Here's how the part is built. I have some questions about the finished solid (model axes, mm). A direction names the side the tool comes from. Round coordinates to 2 decimals unless told otherwise and drop trailing zeros. Order: outer loops, then holes, each group sorted by start corner. A loop starts at its lowest first (then second) coordinate and runs counter-clockwise, first axis right, second up. Notation, with made-up numbers: M -27.5,-31.5 L 25.5,-31.5 A22 cw 25.5,-1.5 Z; hole C 1.25,13 d11. An arc over 180 degrees is marked long. Write item = value, one per line. Start each with the question number.
Item 1: We'd pull the mould along Y, two halves only. Please class faces 1 (the face through (20.95, 4.035, 18.483)), 2 (the face through (-16, -3.204, 11)), 3 (the face through (-28, -1, 23)): pulls with the +Y half, pulls with the -Y half, needs draft (parallel to the pull), parting line crosses it, or undercut.
Item 2: I'm going to push flat-ended pins straight in: P1, Ø2, axis at x = -27, z = 12.5, coming from the +Y side; P2, Ø2, axis at x = -16, y = -0.5, coming from the +Z side; P3, Ø1.5, axis at x = -19.5, z = 3.5, coming from the -Y side; P4, Ø1.5, axis at x = 14.5, z = 8.5, coming from the -Y side. Where does each tip first touch, or does it pass through?
Item 3: I want a section at C-C, the plane x = -19.5. List the corners of the cut face in (y, z) for me, plus the area to 3 significant figures.
Item 4: I want a section at A-A, the plane z = 16.5. State how many separate pieces and enclosed holes the cut face has, plus the area to 3 significant figures.
Item 5: I want a section at D-D, the plane y = 17.5. List the corners of the cut face in (x, z) for me, plus the area to 3 significant figures.
Item 6: For faces 4 (the face through (17.436, 23.244, 13.797)), 5 (the face through (-28, 5.796, 16)), 6 (the face through (-24.831, 12, 12)), 7 (the face through (-28, 26.796, 12)), which set-ups out of +Z, -Z, +X, -X, +Y, -Y let a thin tool reach every point of the face, with its end or its side?
Item 7: Please list where these lines run through material, in increasing order: L1, parallel to X at y = 24, z = 9.25; L2, parallel to X at y = 19, z = 9; L3, parallel to X at y = 19.5, z = 15.25.
```python
from build123d import *

# Parameters (mm, degrees)
SKETCH1_W            = 7
SKETCH1_H            = 29
SIDES_DEPTH          = 23
SIDES_2_DEPTH        = 23
BACK_PLATE_DEPTH     = 2
SKETCH2_W            = 32
SKETCH2_H            = 27
BEARING_BASE_DEPTH   = 1
SKETCH3_W            = 14.5
SKETCH3_H            = 6
WIRE_2_DEPTH         = 21
BEARING_START        = 1
BEARING_DEPTH        = 7.5
MOUTNING_HOLES_R     = 2
SCREW_HOLES_DEPTH    = 10
SCREW_START          = -4.5
MOUTNING_HOLES_3_R   = 4
MOUTNING_HOLES_3_R_2 = 2
SCREW_HEADS_DEPTH    = 2.5


# Read off the part's stored shape, not the designer's step: Bearing
with BuildPart() as part:
    # Sketch1 → Sides (new body)
    with BuildSketch(Plane.XY):
        with Locations((-28.331246011, 12.295832375)):
            Rectangle(SKETCH1_W, SKETCH1_H)
    extrude(amount=SIDES_DEPTH)



with BuildPart() as body_2:
    # Sketch1 → Sides 2 (new body)
    with BuildSketch(Plane.XY):
        with Locations((19.668753989, 12.295832375)):
            Rectangle(SKETCH1_W, SKETCH1_H)
    extrude(amount=SIDES_2_DEPTH)


with BuildPart() as part_1:
    add(part.part)

    add(body_2.part)  # Back Plate merges body 2
    # Sketch1<3> → Back Plate (add)
    with BuildSketch(Plane.XY):
        Polygon((-4.331246011, -2.204167625), (-4.331246011, 34.795832375), (-31.831246011, 34.795832375), (-31.831246011, 26.795832375), (-24.831246011, 26.795832375), (-24.831246011, -2.204167625), align=None)
        Polygon((23.168753989, 34.795832375), (-4.331246011, 34.795832375), (-4.331246011, -2.204167625), (16.168753989, -2.204167625), (16.168753989, 26.795832375), (23.168753989, 26.795832375), align=None)
    extrude(amount=BACK_PLATE_DEPTH)

    # Sketch2 → Bearing Base (add)
    with BuildSketch(Plane.XZ.offset(2.204167625)):
        with Locations((-15.831246011, 13.5)):
            Rectangle(SKETCH2_W, SKETCH2_H)
    extrude(amount=BEARING_BASE_DEPTH)

    # Sketch3 → Wire 2 (cut)
    with BuildSketch(Plane.ZY.offset(31.831246011)):
        with Locations((15.75, 2.795832375)):
            Rectangle(SKETCH3_W, SKETCH3_H)
    extrude(amount=-WIRE_2_DEPTH, mode=Mode.SUBTRACT)

    # Bearing outline → Bearing (add)
    with BuildSketch(Plane.XZ.offset(2.204167625).offset(BEARING_START)):
        with BuildLine():
            Line((-31.831246011, 27), (-31.831246011, 0))
            Line((-31.831246011, 0), (-18.189741294, 0))
            ThreePointArc((-18.189741294, 0), (-15.831246011, 22.25), (-13.472750728, 0))
            Line((-13.472750728, 0), (0.168753989, 0))
            Line((0.168753989, 0), (0.168753989, 27))
            Line((0.168753989, 27), (-31.831246011, 27))
        make_face()
    extrude(amount=BEARING_DEPTH)

    # Moutning Holes → Screw Holes (cut)
    with BuildSketch(Plane(origin=(23.168753989, 0, 0), x_dir=(0, 0, -1), z_dir=(1, 0, 0))):
        with Locations(Location((-6.5, 4.295832375, 0), (0, 0, 90))):
            Circle(MOUTNING_HOLES_R)
        with Locations(Location((-16.5, 4.295832375, 0), (0, 0, 90))):
            Circle(MOUTNING_HOLES_R)
        with Locations(Location((-16.5, 20.295832375, 0), (0, 0, 90))):
            Circle(MOUTNING_HOLES_R)
        with Locations(Location((-6.5, 20.295832375, 0), (0, 0, 90))):
            Circle(MOUTNING_HOLES_R)
    extrude(amount=-SCREW_HOLES_DEPTH, mode=Mode.SUBTRACT)

    # Moutning Holes<3> → Screw Heads (cut)
    # profile 1 of 4: a face of its own
    with BuildSketch(Plane(origin=(23.168753989, 0, 0), x_dir=(0, 0, -1), z_dir=(1, 0, 0)).offset(SCREW_START)):
        with Locations(Location((-6.5, 4.295832375, 0), (0, 0, 270))):
            Circle(MOUTNING_HOLES_3_R)
        with Locations(Location((-6.5, 4.295832375, 0), (0, 0, 90))):
            Circle(MOUTNING_HOLES_3_R_2, mode=Mode.SUBTRACT)
    # profile 2 of 4: a face of its own
    with BuildSketch(Plane(origin=(23.168753989, 0, 0), x_dir=(0, 0, -1), z_dir=(1, 0, 0)).offset(SCREW_START)):
        with Locations(Location((-16.5, 4.295832375, 0), (0, 0, 270))):
            Circle(MOUTNING_HOLES_3_R)
        with Locations(Location((-16.5, 4.295832375, 0), (0, 0, 90))):
            Circle(MOUTNING_HOLES_3_R_2, mode=Mode.SUBTRACT)
    # profile 3 of 4: a face of its own
    with BuildSketch(Plane(origin=(23.168753989, 0, 0), x_dir=(0, 0, -1), z_dir=(1, 0, 0)).offset(SCREW_START)):
        with Locations(Location((-16.5, 20.295832375, 0), (0, 0, 270))):
            Circle(MOUTNING_HOLES_3_R)
        with Locations(Location((-16.5, 20.295832375, 0), (0, 0, 90))):
            Circle(MOUTNING_HOLES_3_R_2, mode=Mode.SUBTRACT)
    # profile 4 of 4: a face of its own
    with BuildSketch(Plane(origin=(23.168753989, 0, 0), x_dir=(0, 0, -1), z_dir=(1, 0, 0)).offset(SCREW_START)):
        with Locations(Location((-6.5, 20.295832375, 0), (0, 0, 270))):
            Circle(MOUTNING_HOLES_3_R)
        with Locations(Location((-6.5, 20.295832375, 0), (0, 0, 90))):
            Circle(MOUTNING_HOLES_3_R_2, mode=Mode.SUBTRACT)
    extrude(amount=-SCREW_HEADS_DEPTH, mode=Mode.SUBTRACT)


solid = part_1.part
```
Filled in:
q1.face_1 = undercut
q1.face_2 = pulls with the -Y half
q1.face_3 = needs draft
q2.P1 = 26.8
q2.P2 = 2
q2.P3 = -3.2
q2.P4 = through
q3.outline = M -10.7,0 L 34.8,0 L 34.8,2 L -2.2,2 L -2.2,27 L -10.7,27 L -10.7,21.63 L -3.2,21.63 L -3.2,0.37 L -10.7,0.37 Z
q3.area = 144 mm^2
q4.separate_pieces = 5
q4.enclosed_holes = 0
q4.area = 413 mm^2
q5.outline = M -31.83,0 L 23.17,0 L 23.17,23 L 16.17,23 L 16.17,19.36 L 18.67,19.36 L 18.67,13.64 L 16.17,13.64 L 16.17,9.36 L 18.67,9.36 L 18.67,3.64 L 16.17,3.64 L 16.17,2 L -24.83,2 L -24.83,23 L -31.83,23 Z
q5.area = 375 mm^2
q6.face_4 = none
q6.face_5 = +Z, -X
q6.face_6 = +Z, +Y
q6.face_7 = +Z, +X, -X, +Y
q7.L1 = -31.83 to -24.83, 16.17 to 23.17
q7.L2 = -31.83 to -24.83, 18.67 to 23.17
q7.L3 = -31.83 to -24.83
